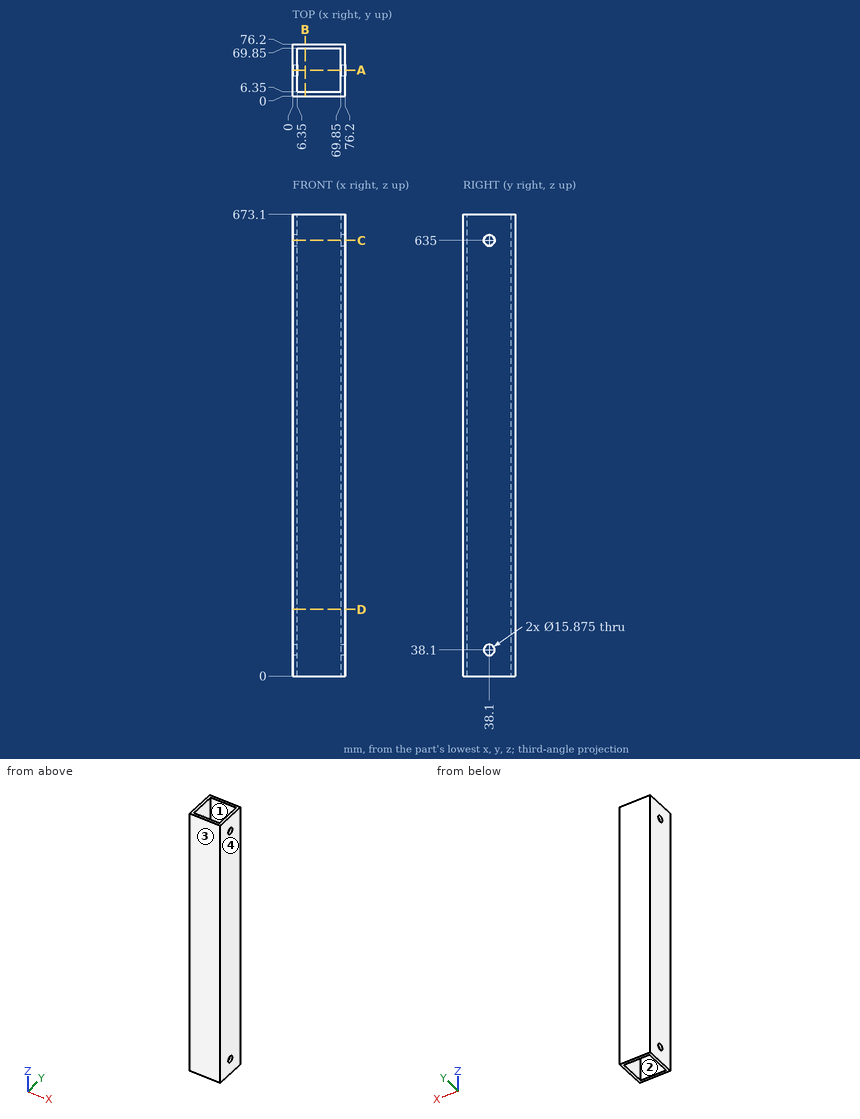
Answer from the drawing. Dimensions are ordinates in mm from the lowest x, y and z of the part. Coordinates: 2 decimals unless noted, no trailing zeros. Order: outer loops, then holes, each group sorted by start corner. A loop starts at its lowest first (then second) coordinate and runs counter-clockwise, first axis right, second up. Notation, with made-up numbers: (-9.5, -16) - (44.5, -16) arc R29 cw to (44.5, 14) - close; hole circle Ø3 at (-8.5, 63.5). An arc over 180 degrees is marked (long way). Answer as a JSON object with one key per item and string values. Group by question number.
Item 1: Section A-A (y = 38.1) is taken. Give the vertices of the cut face in (x, z), plus the area to 3 significant figures.
Item 2: Section D-D (z = 97) is taken. Give the vertices of the cut face in (x, y), plus the area to 3 significant figures.
Item 3: The mould has two halves that part along X. Classify the marked faces 1, 2, 3 and 4: +X half, -X half, draft (parallel to the pull), parting line (faces both ways), or undercut.
Item 4: Section C-C (z = 635) is taken. Give the vertices of the cut face in (x, y).
Item 5: Flat-ended cylindrical pins translate along their axes: P1, Ø19, axis at x = 36.5, z = 211.5, coming from the -Y side; P2, Ø12.5, axis at y = 38.1, z = 38.1, coming from the +X side. Find the tip coordinate at first contact, or state that the pin passes through.
Item 6: Section B-B (x = 18) is taken. Give the vertices of the cut face in (y, z), plus the area to 3 significant figures.
Item 7: Consider probe 1 along Z at (x, y) = (3, 38); probe 2 along X at (y, z) = (21.5, 40). Determine where each line is inside the solid, lowest interval first. Write a range as from..to.
Results are:
{
 "1": {"outline": "(0, 0) - (6.35, 0) - (6.35, 30.16) - (0, 30.16) - close; (0, 46.04) - (6.35, 46.04) - (6.35, 627.06) - (0, 627.06) - close; (0, 642.94) - (6.35, 642.94) - (6.35, 673.1) - (0, 673.1) - close; (69.85, 0) - (76.2, 0) - (76.2, 30.16) - (69.85, 30.16) - close; (69.85, 46.04) - (76.2, 46.04) - (76.2, 627.06) - (69.85, 627.06) - close; (69.85, 642.94) - (76.2, 642.94) - (76.2, 673.1) - (69.85, 673.1) - close", "area": "8,150 mm^2"},
 "2": {"outline": "(0, 0) - (76.2, 0) - (76.2, 76.2) - (0, 76.2) - close; hole (6.35, 6.35) - (69.85, 6.35) - (69.85, 69.85) - (6.35, 69.85) - close", "area": "1,770 mm^2"},
 "3": {"face 1": "undercut", "face 2": "undercut", "face 3": "draft", "face 4": "+X half"},
 "4": {"outline": "(0, 0) - (76.2, 0) - (76.2, 30.16) - (69.85, 30.16) - (69.85, 6.35) - (6.35, 6.35) - (6.35, 30.16) - (0, 30.16) - close; (0, 46.04) - (6.35, 46.04) - (6.35, 69.85) - (69.85, 69.85) - (69.85, 46.04) - (76.2, 46.04) - (76.2, 76.2) - (0, 76.2) - close"},
 "5": {"P1": "stops at y = 0", "P2": "passes through"},
 "6": {"outline": "(0, 0) - (6.35, 0) - (6.35, 673.1) - (0, 673.1) - close; (69.85, 0) - (76.2, 0) - (76.2, 673.1) - (69.85, 673.1) - close", "area": "8,550 mm^2"},
 "7": {"probe 1": "z = 0..30.16, 46.04..627.06, 642.94..673.1", "probe 2": "x = 0..6.35, 69.85..76.2"}
}
